For this review, use the dimensioned drawing (mm, ordinates from the lowest corner) and the shaded views. Round coordinates to 2 decimals unless told otherwise and drop trailing zeros. Write each loop counter-clockwise with the first axis right and the second up, starting at its lowest first coordinate (ties: lowest second). Pieces come first, ordered by that corner, then holes. Notation, with made-up numbers: M 22.5,10.25 L 30.5,10.25 A27 cw 30.5,31.25 Z; hole C 83,-18 d8. An arc over 180 degrees is marked long. Use one line per item in the form item = value. Start each with the question number.
Item 1: Add section A-A (x = 24.5). State the section outline as (y, z) points.
Item 2: Add section B-B (y = 1.3). State the section outline as (x, z) points, and give its area (3 significant figures).
Item 3: For line 1 (Z direction, x = 24.5, y = 1.2); line 2 (X direction, y = 0.9, z = 32.75); line 3 (Z direction, x = 41.5, y = 1.05), list the stretches that pass through material, from the lowest coordinate up. Write a range as [from, to].
Item 4: For P1, Ø1, axis at y = 1.5, z = 6.5, coming from the +X side; P2, Ø1, axis at x = 42.5, y = 1, coming from the +Z side; P3, Ø1, axis at y = 1, z = 6.5, coming from the -X side, all flat-tipped, find the tip position at first contact; note any pin that passes through.
Item 5: Add section C-C (x = 33). State the section outline as (y, z) points, and give its area (3 significant figures).
Item 6: Add section D-D (z = 8.5). State the section outline as (x, y) points.
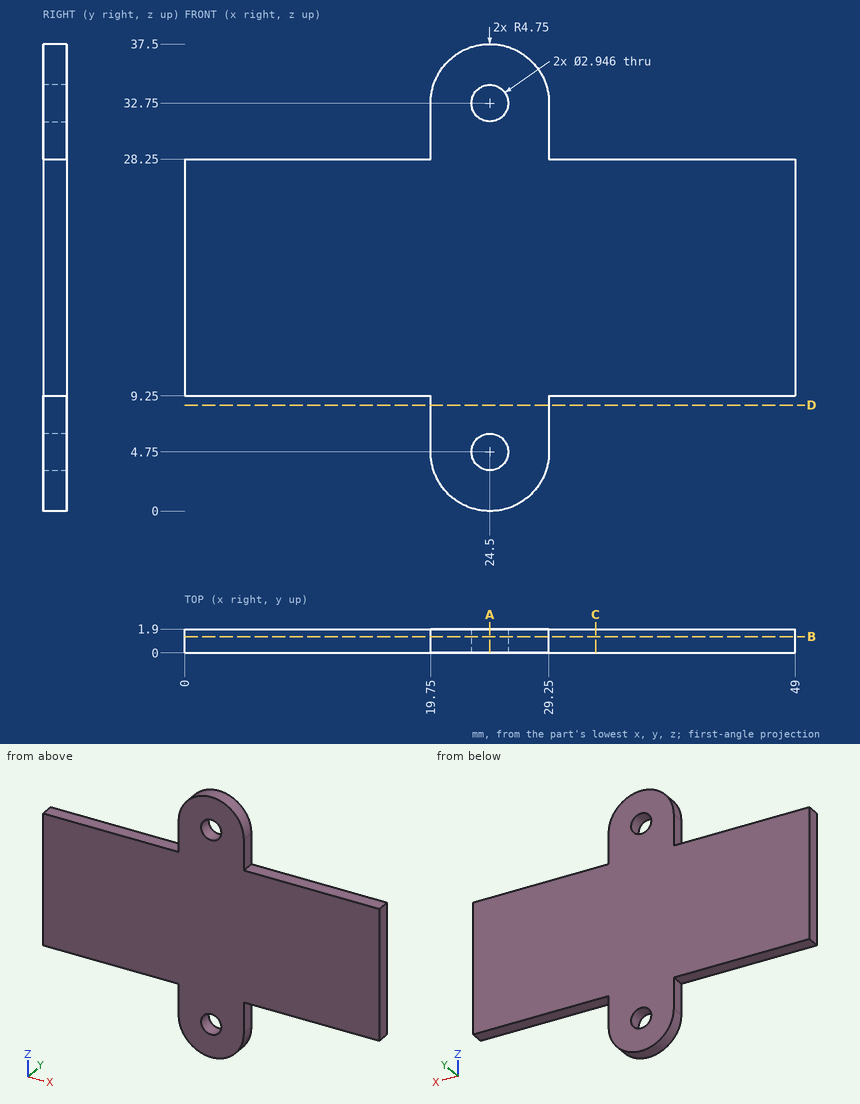
Calculated:
q1.outline = M 0,0 L 1.9,0 L 1.9,3.28 L 0,3.28 Z; M 0,6.22 L 1.9,6.22 L 1.9,31.28 L 0,31.28 Z; M 0,34.22 L 1.9,34.22 L 1.9,37.5 L 0,37.5 Z
q2.outline = M 0,9.25 L 19.75,9.25 L 19.75,4.75 A4.75 ccw 29.25,4.75 L 29.25,9.25 L 49,9.25 L 49,28.25 L 29.25,28.25 L 29.25,32.75 A4.75 ccw 19.75,32.75 L 19.75,28.25 L 0,28.25 Z; hole C 24.5,4.75 d2.95; hole C 24.5,32.75 d2.95
q2.area = 1,070 mm^2
q3.line_1 = [0, 3.28], [6.22, 31.28], [34.22, 37.5]
q3.line_2 = [19.75, 23.03], [25.97, 29.25]
q3.line_3 = [9.25, 28.25]
q4.P1 = 29.25
q4.P2 = 28.25
q4.P3 = 19.75
q5.outline = M 0,9.25 L 1.9,9.25 L 1.9,28.25 L 0,28.25 Z
q5.area = 36.1 mm^2
q6.outline = M 19.75,0 L 29.25,0 L 29.25,1.9 L 19.75,1.9 Z
